Check sheet for the modelled part. Datum: model origin and axes. Units: mm. Round coordinates to 2 decimals unless told otherwise and drop trailing zeros. Loops run counter-clockwise (first coordinate to the right, second up) from the corner with the lowest first, then second, coordinate; pieces in that order, holes last. Notation, with made-up numbers: (0, 24.25) -> (39, 24.25) arc R7 cw to (39, 36.25) -> close; hole circle Ø8 at (-31, 50). An arc over 180 degrees is marked (long way). Return JSON: item names as keys, results as strings.
from build123d import *

# Parameters (mm, degrees)
SKETCH2_R           = 3.5
BOSS_EXTRUDE1_DEPTH = 6
SKETCH3_R           = 2.475
CUT_EXTRUDE1_DEPTH  = 2.5
BOSS_EXTRUDE2_DEPTH = 3


with BuildPart() as part:
    # Sketch2 → Boss-Extrude1 (new body)
    with BuildSketch(Plane(origin=(0, 0, 0), x_dir=(1, 0, 0), z_dir=(0, 1, 0))):
        Circle(SKETCH2_R)
    extrude(amount=BOSS_EXTRUDE1_DEPTH)

    # Sketch3 → Cut-Extrude1 (cut)
    with BuildSketch(Plane.XZ):
        Circle(SKETCH3_R)
    extrude(amount=-CUT_EXTRUDE1_DEPTH, mode=Mode.SUBTRACT)

    # Sketch4 → Boss-Extrude2 (add)
    with BuildSketch(Plane(origin=(0, 6, 0), x_dir=(1, 0, 0), z_dir=(0, 1, 0))):
        with BuildLine():
            Line((0, 3.5), (20, 3.5))
            Line((20, 3.5), (20, -3.5))
            Line((20, -3.5), (0, -3.5))
            ThreePointArc((0, -3.5), (3.5, 0), (0, 3.5))
        make_face()
    extrude(amount=-BOSS_EXTRUDE2_DEPTH)


solid = part.part
Q1. Section check C-C (x = 7.25). Record the boundary of the cut face in (y, z).
Results list:
{"outline": "(3, -3.5) -> (6, -3.5) -> (6, 3.5) -> (3, 3.5) -> close"}
Q2. Draft check along Z on faces 1 (the flat face through (10, 5, -3.5)), 2 (the flat face through (0, 2.5, 0)), 3 (the cylindrical face through (-3.497, 2.291, -0.154)), 4 (the cylindrical face through (2.36, 1.23, 0.74)). Enter one of: released by +Z, released by -Z, zero draft, split by the parting line, or undercut.
Results list:
{"face 1": "released by -Z", "face 2": "undercut", "face 3": "split by the parting line", "face 4": "undercut"}
Q3. Section check D-D (z = -1.5). Record the boundary of the cut face in (x, y), then the cut area to 3 significant figures.
Results list:
{"outline": "(-3.16, 0) -> (-1.97, 0) -> (-1.97, 2.5) -> (1.97, 2.5) -> (1.97, 0) -> (3.16, 0) -> (3.16, 3) -> (20, 3) -> (20, 6) -> (-3.16, 6) -> close", "area": "78.6 mm^2"}
Q4. Section check A-A (z = 0). Record the boundary of the cut face in (x, y) (3 decimals).
Results list:
{"outline": "(-3.5, 0) -> (-2.475, 0) -> (-2.475, 2.5) -> (2.475, 2.5) -> (2.475, 0) -> (3.5, 0) -> (3.5, 3) -> (20, 3) -> (20, 6) -> (-3.5, 6) -> close"}
Q5. Section check B-B (y = 4.2). Record the boundary of the cut face in (x, z).
Results list:
{"outline": "(0, -3.5) -> (20, -3.5) -> (20, 3.5) -> (0, 3.5) arc R3.5 ccw to start"}
Q6. Material ranges on line 1 (Z direction, x = 0, y = 2) (3 decimals); line 2 (Y direction, x = -0.75, z = -0.25); line 3 (Y direction, x = 16.25, z = -0.25), recorded low to high.
Results list:
{"line 1": "-3.5 to -2.475, 2.475 to 3.5", "line 2": "2.5 to 6", "line 3": "3 to 6"}
Q7. Go/stop test with a flat-tipped pin: pin 1 (2.5 mm diameter, centred on x = 0.5, z = 0.5, fed in from -Y). Record where the tip stops, or that it passes through.
Results list:
{"pin 1": "y = 2.5"}
